from build123d import *

# Parameters (mm, degrees)
SKETCH1_R              = 3.175
BOSS_EXTRUDE1_DEPTH    = 6.35
FILLET1_R              = 3.175
F_10_CLEARANCE_HOLE1_D = 5.1054


with BuildPart() as part:
    # Sketch1 → Boss-Extrude1 (new body)
    with BuildSketch(Plane(origin=(0, 0, 0), x_dir=(1, 0, 0), z_dir=(0, 1, 0))):
        with BuildLine():
            ThreePointArc((55.88, 63.5), (0, 7.62), (-55.88, 63.5))
            Line((-55.88, 63.5), (-65.405, 63.5))
            Line((-65.405, 63.5), (-101.231750934, -37.066318412))
            ThreePointArc((-101.231750934, -37.066318412), (-101.50726052, -38.116025925), (-101.6, -39.197317183))
            Line((-101.6, -39.197317183), (-101.6, -63.5))
            Line((-101.6, -63.5), (101.6, -63.5))
            Line((101.6, -63.5), (101.6, -39.197317183))
            ThreePointArc((101.6, -39.197317183), (101.50726052, -38.116025925), (101.231750934, -37.066318412))
            Line((101.231750934, -37.066318412), (65.405, 63.5))
            Line((65.405, 63.5), (55.88, 63.5))
        make_face()
        with Locations(Location((-63.5, -50.8, 0), (0, 0, 270))):
            Circle(SKETCH1_R, mode=Mode.SUBTRACT)
        with Locations(Location((-25.4, -50.8, 0), (0, 0, 270))):
            Circle(SKETCH1_R, mode=Mode.SUBTRACT)
        with BuildLine():
            Line((-30.492459165, -38.1), (-82.485514384, -38.1))
            ThreePointArc((-82.485514384, -38.1), (-87.67465411, -35.409962965), (-88.467265319, -29.61900123))
            Line((-88.467265319, -29.61900123), (-67.620951247, 28.896968093))
            ThreePointArc((-67.620951247, 28.896968093), (-62.60882158, 33.04150393), (-56.579551543, 30.602954379))
            Line((-56.579551543, 30.602954379), (-24.890648803, -28.759645393))
            ThreePointArc((-24.890648803, -28.759645393), (-25.046761241, -35.016018084), (-30.492459165, -38.1))
        make_face(mode=Mode.SUBTRACT)
        with BuildLine():
            ThreePointArc((-5.299041163, -38.1), (-8.565059247, -37.195697924), (-10.900851525, -34.740354607))
            Line((-10.900851525, -34.740354607), (-24.84623891, -8.616557995))
            ThreePointArc((-24.84623891, -8.616557995), (-24.197984845, -1.653196967), (-17.541381774, 0.491159744))
            ThreePointArc((-17.541381774, 0.491159744), (-0.588821605, -1.902349454), (16.404084946, 0.185546499))
            ThreePointArc((16.404084946, 0.185546499), (22.928583423, -1.961591642), (23.68255589, -8.788802499))
            Line((23.68255589, -8.788802499), (10.859081809, -34.577314678))
            ThreePointArc((10.859081809, -34.577314678), (8.517567892, -37.14796018), (5.173240471, -38.1))
            Line((5.173240471, -38.1), (-5.299041163, -38.1))
        make_face(mode=Mode.SUBTRACT)
        with Locations(Location((25.4, -50.8, 0), (0, 0, 270))):
            Circle(SKETCH1_R, mode=Mode.SUBTRACT)
        with Locations(Location((63.5, -50.8, 0), (0, 0, 270))):
            Circle(SKETCH1_R, mode=Mode.SUBTRACT)
        with BuildLine():
            Line((67.620951247, 28.896968093), (88.467265319, -29.61900123))
            ThreePointArc((88.467265319, -29.61900123), (87.67465411, -35.409962965), (82.485514384, -38.1))
            Line((82.485514384, -38.1), (29.423726477, -38.1))
            ThreePointArc((29.423726477, -38.1), (23.956198754, -34.979340583), (23.862621229, -28.684611212))
            Line((23.862621229, -28.684611212), (56.428690976, 30.395444829))
            ThreePointArc((56.428690976, 30.395444829), (62.481851802, 33.059810636), (67.620951247, 28.896968093))
        make_face(mode=Mode.SUBTRACT)
    extrude(amount=BOSS_EXTRUDE1_DEPTH)

    # Fillet1
    fillet1_edges = [part.edges().sort_by_distance(p)[0] for p in [
        (-65.405, 3.175, -63.5),
        (65.405, 3.175, -63.5),
    ]]
    fillet(fillet1_edges, radius=FILLET1_R)

    # #10 Clearance Hole1 (through all)
    with Locations(Plane(origin=(0, 6.35, 0), x_dir=(1, 0, 0), z_dir=(0, 1, 0))):
        with Locations((52.959, -50.8), (88.9, -50.8)):
            Hole(F_10_CLEARANCE_HOLE1_D / 2)


solid = part.part
The listing builds one solid part. Answer for the finished solid, in the listing's coordinates (mm). A direction names the side the tool comes from. Round coordinates to 2 decimals unless told otherwise and drop trailing zeros. Order: outer loops, then holes, each group sorted by start corner. A loop starts at its lowest first (then second) coordinate and runs counter-clockwise, first axis right, second up. Notation, with made-up numbers: M -22,32.5 L 37,32.5 A24 cw 37,68.5 Z; hole C 81.25,61.25 d7. An arc over 180 degrees is marked long. Answer in a Markdown table with one row per item. Add a question column.
1) Consider line 1 along X through (y, z) = (0.5, 24.5) (3 decimals); line 2 along X through (y, z) = (1.5, 15.5); line 3 along Z through (x, y) = (43, 5.5). Determine where each line is inside the solid, lowest interval first. Write a range as from..to.
2) Which of the six approach directions +Z, -Z, +X, -X, +Y, -Y give full straight-line access (tool end or side, diameter ignored) to faces 1 (the face through (-101.6, 3, 51)), 2 (the face through (-78.2, 3.1, 0.8))?
3) The part is cut by section A-A on z = 50.8. Determine the outline of the cut face in (x, y) (3 decimals).
4) The part is cut by section C-C on y = 3.75. Count the separate pieces of the cut face and the enclosed holes in it, plus the area to 3 significant figures.
5) Determine the mould class of faces 3 (the face through (101.6, 3, 52)), 4 (the face through (60, 3, -63.5)), 5 (the face through (87.723, 3.131, 35.34)) for opening direction Z: pulls with the +Z half, pulls with the -Z half, needs draft (parallel to the pull), parting line crosses it, or undercut.
6) The part is cut by section B-B on x = -76. Determine the outline of the cut face in (y, z).
7) Flat-ended cylindrical pins translate along their axes: pin 1 Ø1.5 at (x, y) = (-6, 4) entering from -Z; pin 2 Ø4 at (x, z) = (25.4, 50.8) entering from -Y; pin 3 Ø1 at (y, z) = (4, -7) entering from -X; pin 4 Ø1.5 at (y, z) = (3, -12) entering from -X. Find the tip coordinate at first contact, or state that the pin passes through.
8) The part is cut by section D-D on x = 8.5. Determine the outline of the cut face in (y, z).
Findings below:
| question | item | result |
|---|---|---|
| 1 | line 1 | x = -96.755..-86.644, -27.165..-16.367, 15.87..26.169, 86.644..96.755 |
| 1 | line 2 | x = -93.55..-83.44, -31.97..-21.17, 20.35..31.13, 83.44..93.55 |
| 1 | line 3 | z = -27.81..-6.03, 38.1..63.5 |
| 2 | face 1 | +Z, -Z, -X, +Y, -Y |
| 2 | face 2 | +Y, -Y |
| 3 | outline | M -101.6,0 L -66.675,0 L -66.675,6.35 L -101.6,6.35 Z; M -60.325,0 L -28.575,0 L -28.575,6.35 L -60.325,6.35 Z; M -22.225,0 L 22.225,0 L 22.225,6.35 L -22.225,6.35 Z; M 28.575,0 L 50.406,0 L 50.406,6.35 L 28.575,6.35 Z; M 55.512,0 L 60.325,0 L 60.325,6.35 L 55.512,6.35 Z; M 66.675,0 L 86.347,0 L 86.347,6.35 L 66.675,6.35 Z; M 91.453,0 L 101.6,0 L 101.6,6.35 L 91.453,6.35 Z |
| 4 | separate pieces | 1 |
| 4 | enclosed holes | 9 |
| 4 | area | 10,100 mm² |
| 5 | face 3 | needs draft |
| 5 | face 4 | pulls with the -Z half |
| 5 | face 5 | undercut |
| 6 | outline | M 0,-33.76 L 6.35,-33.76 L 6.35,-5.38 L 0,-5.38 Z; M 0,38.1 L 6.35,38.1 L 6.35,63.5 L 0,63.5 Z |
| 7 | pin 1 | stops at z = -8.03 |
| 7 | pin 2 | passes through |
| 7 | pin 3 | stops at x = -85.71 |
| 7 | pin 4 | stops at x = -84.02 |
| 8 | outline | M 0,-8.27 L 6.35,-8.27 L 6.35,1.35 L 0,1.35 Z; M 0,37.16 L 6.35,37.16 L 6.35,63.5 L 0,63.5 Z |
